Work out the finished part from the listing and answer in its coordinate system (mm). Face numbers are marked on the shaded views. Give positions to 0.01 mm unless a question says otherwise; leave off trailing zeros. Write each loop counter-clockwise with the first axis right and the second up, starting at its lowest first coordinate (ties: lowest second). Pieces come first, ordered by that corner, then holes.
1) Find section D-D (y = 8.7). Determine the outline of the cut face in (x, z), plus the area to 3 significant figures.
2) Straight lines are drawn through the part: probe 1 along Y at (x, z) = (-2, -0.95); probe 2 along Y at (x, z) = (0.25, -2.8); probe 3 along X at (y, z) = (-14.7, -0.2). For each, find the intervals that lie inside material, in ascending order.
3) Find section A-A (z = -0.05). Count the separate pieces of the cut face and the enclosed holes in it, plus the area to 3 significant figures.
4) Find section B-B (y = -6.7). Determine the outline of the cut face in (x, z), plus the area to 3 significant figures.
5) Given pin 1 Ø1.6 at (x, y) = (0, 14.7) entering from -Z; pin 2 Ø1 at (x, z) = (-0.5, -2.5) entering from -Y; pin 3 Ø1.5 at (x, z) = (2, -2.5) entering from +Y, each flat-ended and moving along its own axis, determine where each tip first touches the part or whether it passes through.
6) Find section C-C (y = -3). Determine the outline of the cut face in (x, z).
7) Determine the mould class of the marked faces 1, 2, 3 and 4 for opening direction Y: pulls with the +Y half, pulls with the -Y half, needs draft (parallel to the pull), parting line crosses it, or undercut.
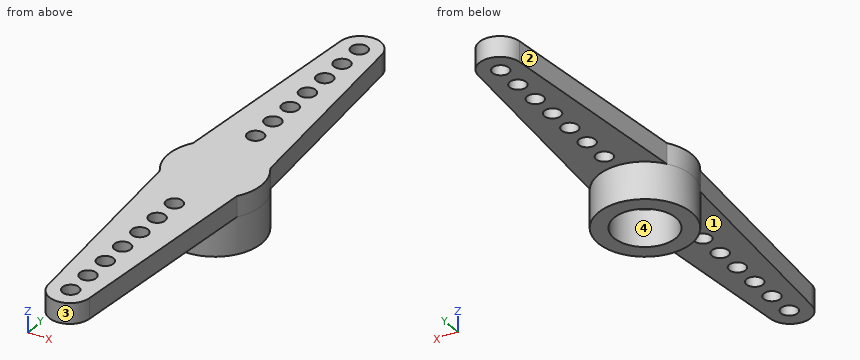
Solid Edge part; units mm, degrees
sketch "Sketch1" plane through (0, 0, 0) normal (0, 0, 1) x (1, 0, 0)
  line L0 (-2.8, 1.9287) -> (-1.4957, 16.9261)
  line L1 (2.8, 1.9287) -> (1.493, 16.9264)
  arc A0 (2.8, 1.9287) -> (2.8, -1.9287) centre (0, 0) cw
  line L2 (2.8, -1.9287) -> (1.493, -16.9264)
  arc A1 (-1.4957, -16.9261) -> (1.493, -16.9264) centre (-0.0013, -16.7962) ccw
  line L3 (-2.8, -1.9287) -> (-1.4957, -16.9261)
  arc A2 (-2.8, -1.9287) -> (-2.8, 1.9287) centre (0, 0) cw
  arc A3 (-1.4957, 16.9261) -> (1.493, 16.9264) centre (-0.0013, 16.7962) cw
  dimension "D1" = 0.0013
extrude "Protrusion1" add sketch "Sketch1" along normal mid plane 1.5
hole "Agujero_8" at (0, 14.7, 2) direction (0, 0, -1) diameter 1.2 end up to next
hole "Hole1" at (0, 4.7, 2) direction (0, 0, -1) diameter 1.2 end up to next
hole "Hole2" at (0, 6.7, 2) direction (0, 0, -1) diameter 1.2 end up to next
hole "Hole3" at (0, 8.7, 2) direction (0, 0, -1) diameter 1.2 end up to next
hole "Hole4" at (0, 10.7, 2) direction (0, 0, -1) diameter 1.2 end up to next
hole "Hole5" at (0, 12.7, 2) direction (0, 0, -1) diameter 1.2 end up to next
hole "Hole6" at (0, 16.7, 2) direction (0, 0, -1) diameter 1.2 end up to next
hole "Hole7" at (0, -14.7, 2) direction (0, 0, -1) diameter 1.2 end up to next
hole "Hole8" at (0, -4.7, 2) direction (0, 0, -1) diameter 1.2 end up to next
hole "Hole9" at (0, -6.7, 2) direction (0, 0, -1) diameter 1.2 end up to next
hole "Hole10" at (0, -8.7, 2) direction (0, 0, -1) diameter 1.2 end up to next
hole "Hole11" at (0, -10.7, 2) direction (0, 0, -1) diameter 1.2 end up to next
hole "Hole12" at (0, -12.7, 2) direction (0, 0, -1) diameter 1.2 end up to next
hole "Hole13" at (0, -16.7, 2) direction (0, 0, -1) diameter 1.2 end up to next
sketch "Sketch2" plane through (0, 7.4481, -0.75) normal (0, 0, -1) x (-0.0868172, 0.9962243, 0)
  circle A0 centre (-7.42, -0.6466) radius 2.25
  circle A1 centre (-7.42, -0.6466) radius 3.4
extrude "ProtrusiónExtruida_2" add sketch "Sketch2" along normal blind 2.7
properties material "ABS, medio impacto"
Results:
1. outline: (-2.21, -0.75) - (-0.6, -0.75) - (-0.6, 0.75) - (-2.21, 0.75) - close; (0.6, -0.75) - (2.21, -0.75) - (2.21, 0.75) - (0.6, 0.75) - close
1. area: 4.83 mm2
2. probe 1: y = -2.75 to -1.03, 1.03 to 2.75
2. probe 2: y = -3.39 to -2.24, 2.24 to 3.39
2. probe 3: x = -1.69 to -0.6, 0.6 to 1.69
3. separate pieces: 1
3. enclosed holes: 14
3. area: 144 mm2
4. outline: (-2.39, -0.75) - (-0.6, -0.75) - (-0.6, 0.75) - (-2.39, 0.75) - close; (0.6, -0.75) - (2.38, -0.75) - (2.38, 0.75) - (0.6, 0.75) - close
4. area: 5.35 mm2
5. pin 1: stops at z = -0.75
5. pin 2: stops at y = -3.4
5. pin 3: stops at y = 3.16
6. outline: (-2.71, -0.75) - (-1.6, -0.75) - (-1.6, -3.45) - (1.6, -3.45) - (1.6, -0.75) - (2.71, -0.75) - (2.71, 0.75) - (-2.71, 0.75) - close
7. face 1: needs draft
7. face 2: pulls with the +Y half
7. face 3: pulls with the -Y half
7. face 4: undercut
